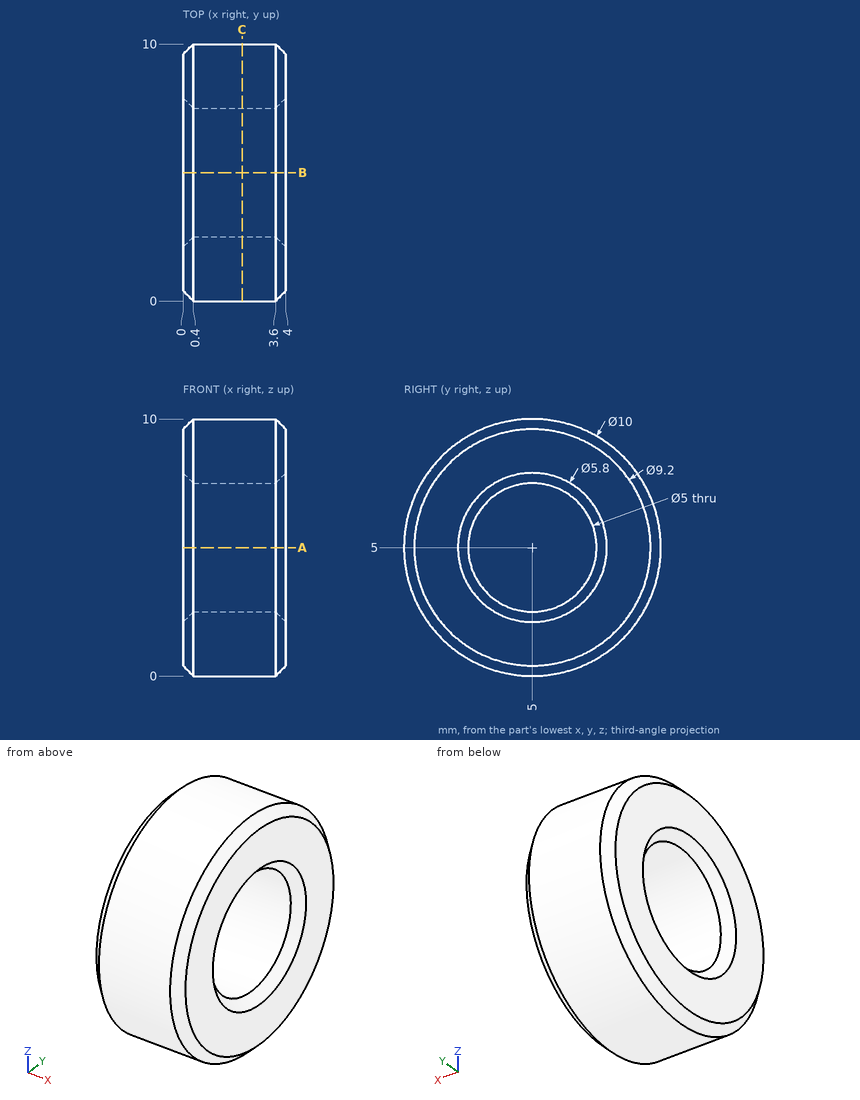
Study the drawing (mm; zero at the part's minimum x, y, z) and answer. Coordinates: 2 decimals unless noted, no trailing zeros. Loops run counter-clockwise (first coordinate to the right, second up) from the corner with the lowest first, then second, coordinate; pieces in that order, holes last. Notation, with made-up numbers: M -12.5,-8 L 34.5,-8 A22 ccw 34.5,29 Z; hole C 65.25,55 d1. An arc over 180 degrees is marked long. Answer in a Markdown table with one row per item. Add a question column.
1. Consider L1, parallel to Y at x = 1.4, z = 5; L2, parallel to Y at x = 1.9, z = 7. Determine where each line is inside the solid, lowest interval first.
2. Find section A-A, the plane z = 5. Write down the section's boundary in (x, y).
3. Find section C-C, the plane x = 2.3. Write down the section's boundary in (y, z), then the cut area to 3 significant figures.
Reported:
| question | item | result |
|---|---|---|
| 1 | L1 | y = 0 to 2.5, 7.5 to 10 |
| 1 | L2 | y = 0.42 to 3.5, 6.5 to 9.58 |
| 2 | outline | M 0,0.4 L 0.4,0 L 3.6,0 L 4,0.4 L 4,2.1 L 3.6,2.5 L 0.4,2.5 L 0,2.1 Z; M 0,7.9 L 0.4,7.5 L 3.6,7.5 L 4,7.9 L 4,9.6 L 3.6,10 L 0.4,10 L 0,9.6 Z |
| 3 | outline | C 5,5 d10; hole C 5,5 d5 |
| 3 | area | 58.9 mm^2 |
